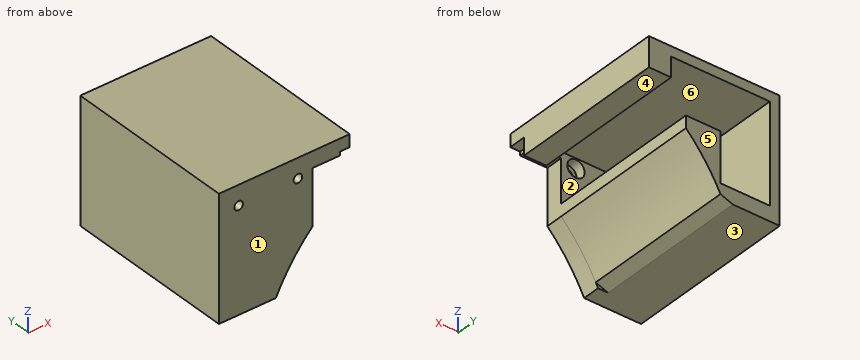
```python
from build123d import *
from build123d.topology import SkipClean

# Parameters (mm, degrees)
SKETCH_1_W          = 50
SKETCH_1_H          = 50
EXTRUDE_1_DEPTH     = 7
SKETCH_2_R          = 80
CUT_EXTRUDE_1_DEPTH = 10
SKETCH_3_W          = 22
SKETCH_3_H          = 30
CUT_EXTRUDE_2_DEPTH = 10
HOLE_WIZARD_1_D     = 3.5
HOLE_WIZARD_2_D     = 7
HOLE_WIZARD_2_DEPTH = 4
EXTRUDE_START       = 63
SKETCH_9_W          = 15
SKETCH_9_H          = 6
SKETCH_9_W_2        = 46
SKETCH_9_H_2        = 4
EXTRUDE_2_DEPTH     = 63
SKETCH_10_W         = 6
SKETCH_10_H         = 8
EXTRUDE_3_DEPTH     = 63
SKETCH_11_W         = 5
SKETCH_11_H         = 1.5
EXTRUDE_4_DEPTH     = 7
EXTRUDE_5_DEPTH     = 3
SKETCH_13_W         = 6
SKETCH_13_H         = 1.5
EXTRUDE_6_DEPTH     = 7
EXTRUDE_7_DEPTH     = 63


with BuildPart() as part:
    # 草图1 → 凸台-拉伸1 (new body)
    with BuildSketch(Plane(origin=(0, 0, 0), x_dir=(1, 0, 0), z_dir=(0, 1, 0))):
        with Locations((25, 25)):
            Rectangle(SKETCH_1_W, SKETCH_1_H)
    extrude(amount=EXTRUDE_1_DEPTH)

    # 草图2 → 切除-拉伸1 (cut)
    with BuildSketch(Plane(origin=(0, 7, 0), x_dir=(1, 0, 0), z_dir=(0, 1, 0))):
        with Locations((95, 85)):
            Circle(SKETCH_2_R)
    extrude(amount=-CUT_EXTRUDE_1_DEPTH, mode=Mode.SUBTRACT)

    # 草图3 → 切除-拉伸2 (cut)
    with BuildSketch(Plane(origin=(0, 7, 0), x_dir=(1, 0, 0), z_dir=(0, 1, 0))):
        with Locations((49, 20)):
            Rectangle(SKETCH_3_W, SKETCH_3_H)
    extrude(amount=-CUT_EXTRUDE_2_DEPTH, mode=Mode.SUBTRACT)

    # 孔1 (through all)
    with Locations(Plane(origin=(0, 0, 0), x_dir=(-1, 0, 0), z_dir=(0, -1, 0))):
        with Locations((-32, 8), (-8, 8)):
            Hole(HOLE_WIZARD_1_D / 2)

    # 孔2
    with Locations(Plane(origin=(0, 7, 0), x_dir=(1, 0, 0), z_dir=(0, 1, 0))):
        with Locations((8, 8), (32, 8)):
            Hole(HOLE_WIZARD_2_D / 2, depth=HOLE_WIZARD_2_DEPTH)

    # 草图9 → 凸台-拉伸2 (add)
    with SkipClean():  # the faces are left unmerged after this step: merging them gives an invalid solid
        with BuildSketch(Plane(origin=(0, 7, 0), x_dir=(1, 0, 0), z_dir=(0, 1, 0)).offset(EXTRUDE_START)):
            with Locations((11.5, 47)):
                Rectangle(SKETCH_9_W, SKETCH_9_H)
            Polygon((0, 50), (0, 0), (4, 0), (4, 4), (4, 44), (4, 50), align=None)
            with Locations((27, 2)):
                Rectangle(SKETCH_9_W_2, SKETCH_9_H_2)
            with BuildLine():
                ThreePointArc((38, 28.866231197), (30.278867045, 37.976867938), (24, 48.135382818))
                Line((24, 48.135382818), (24, 24))
                Line((24, 24), (38, 24))
                Line((38, 24), (38, 28.866231197))
            make_face()
        extrude(amount=-EXTRUDE_2_DEPTH)

    # 草图10 → 凸台-拉伸3 (add)
    with SkipClean():  # the faces are left unmerged after this step: merging them gives an invalid solid
        with BuildSketch(Plane(origin=(0, 7, 0), x_dir=(1, 0, 0), z_dir=(0, 1, 0))):
            with Locations((47, 8)):
                Rectangle(SKETCH_10_W, SKETCH_10_H)
        extrude(amount=EXTRUDE_3_DEPTH)

    # 草图11 → 凸台-拉伸4 (add)
    with SkipClean():  # the faces are left unmerged after this step: merging them gives an invalid solid
        with BuildSketch(Plane.XZ.offset(-7)):
            with Locations((46.5, -5.75)):
                Rectangle(SKETCH_11_W, SKETCH_11_H)
        extrude(amount=EXTRUDE_4_DEPTH)

    # 草图12 → 凸台-拉伸5 (add)
    with SkipClean():  # the faces are left unmerged after this step: merging them gives an invalid solid
        with BuildSketch(Plane(origin=(50, 0, 0), x_dir=(0, 0, -1), z_dir=(1, 0, 0))):
            Polygon((5, 7), (12, 7), (12, 70), (0, 70), (0, 0), (5, 0), align=None)
        extrude(amount=EXTRUDE_5_DEPTH)

    # 草图13 → 凸台-拉伸6 (add)
    with SkipClean():  # the faces are left unmerged after this step: merging them gives an invalid solid
        with BuildSketch(Plane(origin=(0, 0, 0), x_dir=(-1, 0, 0), z_dir=(0, -1, 0))):
            with Locations((-41, 5.75)):
                Rectangle(SKETCH_13_W, SKETCH_13_H)
        extrude(amount=-EXTRUDE_6_DEPTH)

    # 草图15 → 凸台-拉伸7 (add)
    with SkipClean():  # the faces are left unmerged after this step: merging them gives an invalid solid
        with BuildSketch(Plane(origin=(0, 7, 0), x_dir=(1, 0, 0), z_dir=(0, 1, 0))):
            Polygon((19, 44), (24, 44), (24, 48.135382818), (19, 50), align=None)
        extrude(amount=EXTRUDE_7_DEPTH)


solid = part.part
```
Geometry check sheet. Reference: the model listing, model coordinates, mm. Face numbers are marked on the shaded views. A direction names the side the tool comes from. Coordinates: 2 decimals unless noted, no trailing zeros. Write each loop counter-clockwise with the first axis right and the second up, starting at its lowest first coordinate (ties: lowest second). Pieces come first, ordered by that corner, then holes. Notation, with made-up numbers: M -10.5,-9 L 4.5,-9 A29 ccw 4.5,24 Z; hole C 47,23 d8. An arc over 180 degrees is marked long. One line per item, written item: value. Start each with the question number.
(1) Tool access check on the marked faces 4, 5 and 6. Record the directions out of +Z, -Z, +X, -X, +Y, -Y that give a thin tool (end or side, any length) a straight path to the whole face; none if there is none.
(2) Release check for a two-part mould opening along Z. For the marked faces 1, 2 and 3 record: released by +Z, released by -Z, zero draft, split by the parting line, or undercut.
(3) Sectioned sample at A-A, the plane x = 8. Enter the section's corners in (y, z), and give its area (4 significant figures).
(4) Sectioned sample at B-B, the plane y = 53. Enter the section's corners in (x, z), and give its area (3 significant figures).
(5) Sectioned sample at D-D, the plane x = 32. Enter the section's corners in (y, z).
(6) Depth check by flat-ended pin: pin 1 (1.5 mm diameter, centred on y = 51, z = -28, fed in from +X); pin 2 (1.2 mm diameter, centred on x = 51.5, y = 4.5, fed in from -Z); pin 3 (3.5 mm diameter, centred on x = 7.5, z = -6.5, fed in from +Y). Enter the tip coordinate at first touch or a pass-through.
(7) Sectioned sample at C-C, the plane x = 45. Enter the section's corners in (y, z), and give its area (4 significant figures).
(8) Scan lines: line 1 along X through (y, z) = (1.85, -8); line 2 along Z through (x, y) = (8, 5.45); line 3 along Z through (x, y) = (8, 2.3). Record each from-to range of solid material in increasing order. Write a range as [from, to].
Filled sheet:
1. face 4: -Z, +X, +Y, -Y
1. face 5: +Z, -Z, +X, -X, +Y
1. face 6: +Y
2. face 1: zero draft
2. face 2: undercut
2. face 3: released by -Z
3. outline: M 0,-50 L 70,-50 L 70,-44 L 7,-44 L 7,-11.5 L 3,-11.5 L 3,-9.75 L 0,-9.75 Z; M 0,-6.25 L 3,-6.25 L 3,-4.5 L 7,-4.5 L 7,-4 L 70,-4 L 70,0 L 0,0 Z
3. area: 941.5 mm²
4. outline: M 0,-50 L 19,-50 L 24,-48.14 A80 cw 38,-28.87 L 38,-24 L 24,-24 L 24,-44 L 4,-44 L 4,-4 L 44,-4 L 44,-12 L 53,-12 L 53,0 L 0,0 Z
4. area: 772 mm²
5. outline: M 0,-35.69 L 70,-35.69 L 70,-24 L 7,-24 L 7,-11.5 L 3,-11.5 L 3,-9.75 L 0,-9.75 Z; M 0,-6.25 L 3,-6.25 L 3,-4.5 L 7,-4.5 L 7,-4 L 70,-4 L 70,0 L 0,0 Z
6. pin 1: x = 38
6. pin 2: z = -5
6. pin 3: y = 3
7. outline: M 0,-6.5 L 7,-6.5 L 7,-12 L 70,-12 L 70,0 L 0,0 Z
7. area: 801.5 mm²
8. line 1: [0, 6.25], [9.75, 30.25], [33.75, 38]
8. line 2: [-50, -11.5], [-4.5, 0]
8. line 3: [-50, -9.75], [-6.25, 0]
